```python
from build123d import *

# Parameters (mm, degrees)
F0_W     = 250
F0_H     = 250
F0_R     = 52.5
F1_DEPTH = 5
F3_DEPTH = 5.001


with BuildPart() as f1:
    # F0 (on Top) → F1 (new body)
    with BuildSketch(Plane.XY):
        Rectangle(F0_W, F0_H)
        Circle(F0_R, mode=Mode.SUBTRACT)
    extrude(amount=F1_DEPTH)

    # F2 (on face) → F3 (cut, through all)
    with BuildSketch(Plane.XY.offset(5)):
        Polygon((0, 125), (-50, 125), (-50, 120), (0, 120), (50, 120), (50, 125), align=None)
        Polygon((-120, 50), (-125, 50), (-125, 0), (-125, -50), (-120, -50), (-120, 0), align=None)
        Polygon((-50, -120), (-50, -125), (0, -125), (50, -125), (50, -120), (0, -120), align=None)
        Polygon((120, -50), (125, -50), (125, 0), (125, 50), (120, 50), (120, 0), align=None)
    extrude(amount=-F3_DEPTH, mode=Mode.SUBTRACT)


solid = f1.part
```
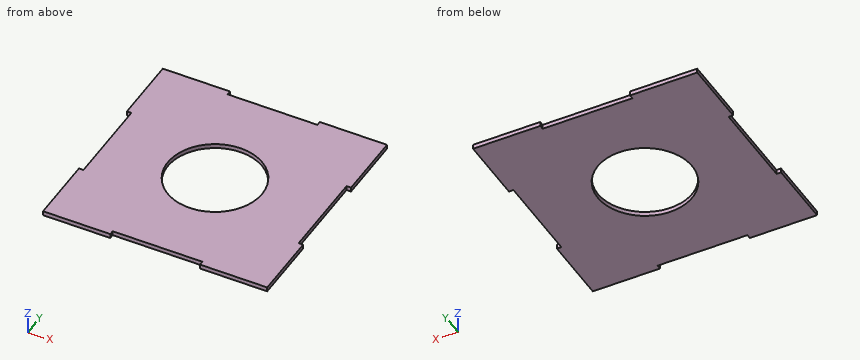
Geometry: final body of the model. Coordinates: model frame, mm. Round coordinates to 2 decimals unless told otherwise and drop trailing zeros. Order: outer loops, then holes, each group sorted by start corner. A loop starts at its lowest first (then second) coordinate and runs counter-clockwise, first axis right, second up. Notation, with made-up numbers: M 72,37.25 L 121,37.25 A5 cw 121,46.25 Z; hole C 22,-16 d2. An arc over 180 degrees is marked long. Use one line per item in the form item = value. Start each with the question number.
Q1. Cut plane A-A (y = 0). Return loops of the section in (x, z).
Q2. Material intervals for line 1 (Y direction, x = 0, z = 3.8); line 2 (Y direction, x = 16, z = 2.85); line 3 (X direction, y = 43, z = 1.75), sorted ascending. Write a range as [from, to].
Q3. Pin query (flat end, axial travel): pin 1 Ø3 at (x, y) = (81.5, -96.5) entering from -Z; pin 2 Ø2.5 at (x, z) = (5.5, 2) entering from -Y; pin 3 Ø12 at (x, y) = (-30.5, -33.5) entering from -Z; pin 4 Ø1.5 at (y, z) = (20.5, 1.5) entering from -X. Return the tip coordinate at first contact, or that it passes through.
Q4. Cut plane C-C (z = 1.15). Return loops of the section in (x, y), and give its area (3 significant figures).
Geometry results:
q1.outline = M -120,0 L -52.5,0 L -52.5,5 L -120,5 Z; M 52.5,0 L 120,0 L 120,5 L 52.5,5 Z
q2.line_1 = [-120, -52.5], [52.5, 120]
q2.line_2 = [-120, -50], [50, 120]
q2.line_3 = [-120, -30.12], [30.12, 120]
q3.pin_1 = 0
q3.pin_2 = -120
q3.pin_3 = through
q3.pin_4 = -120
q4.outline = M -125,-125 L -50,-125 L -50,-120 L 50,-120 L 50,-125 L 125,-125 L 125,-50 L 120,-50 L 120,50 L 125,50 L 125,125 L 50,125 L 50,120 L -50,120 L -50,125 L -125,125 L -125,50 L -120,50 L -120,-50 L -125,-50 Z; hole C 0,0 d105
q4.area = 51,800 mm^2
